Answer from the drawing. Dimensions are ordinates in mm from the lowest x, y and z of the part. Coordinates: 2 decimals unless noted, no trailing zeros. Write each loop counter-clockwise with the first axis right and the second up, starting at its lowest first coordinate (ties: lowest second). Pieces come first, ordered by that corner, then holes. Notation, with made-up numbers: M 17.5,69 L 39.5,69 A15 cw 39.5,85 Z; hole C 49,34.25 d6. An arc over 180 degrees is marked long. Put each result on its own line as item: value. Start each with the question number.
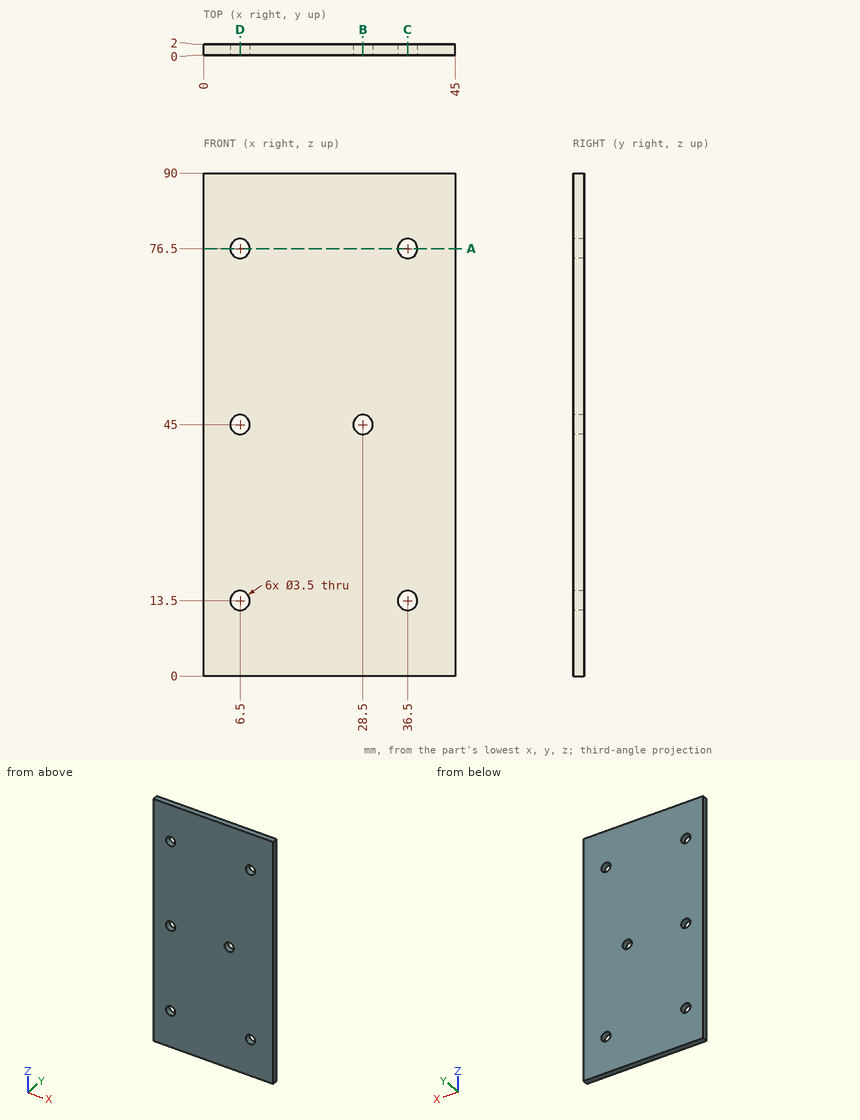
1) Straight lines are drawn through the part: probe 1 along Z at (x, y) = (6.5, 1.25); probe 2 along Z at (x, y) = (36.5, 0.3); probe 3 along X at (y, z) = (1.2, 76.5). For each, find the intervals that lie inside material, in ascending order.
2) A cutting plane is placed at D-D on x = 6.5. Write down the section's boundary in (y, z).
3) A cutting plane is placed at C-C on x = 36.5. Write down the section's boundary in (y, z), then the cut area to 3 significant figures.
4) A cutting plane is placed at A-A on z = 76.5. Write down the section's boundary in (x, y), then the cut area to 3 significant figures.
5) A cutting plane is placed at B-B on x = 28.5. Write down the section's boundary in (y, z), then the cut area to 3 significant figures.
Answers follow:
1. probe 1: z = 0 to 11.75, 15.25 to 43.25, 46.75 to 74.75, 78.25 to 90
1. probe 2: z = 0 to 11.75, 15.25 to 74.75, 78.25 to 90
1. probe 3: x = 0 to 4.75, 8.25 to 34.75, 38.25 to 45
2. outline: M 0,0 L 2,0 L 2,11.75 L 0,11.75 Z; M 0,15.25 L 2,15.25 L 2,43.25 L 0,43.25 Z; M 0,46.75 L 2,46.75 L 2,74.75 L 0,74.75 Z; M 0,78.25 L 2,78.25 L 2,90 L 0,90 Z
3. outline: M 0,0 L 2,0 L 2,11.75 L 0,11.75 Z; M 0,15.25 L 2,15.25 L 2,74.75 L 0,74.75 Z; M 0,78.25 L 2,78.25 L 2,90 L 0,90 Z
3. area: 166 mm²
4. outline: M 0,0 L 4.75,0 L 4.75,2 L 0,2 Z; M 8.25,0 L 34.75,0 L 34.75,2 L 8.25,2 Z; M 38.25,0 L 45,0 L 45,2 L 38.25,2 Z
4. area: 76.0 mm²
5. outline: M 0,0 L 2,0 L 2,43.25 L 0,43.25 Z; M 0,46.75 L 2,46.75 L 2,90 L 0,90 Z
5. area: 173 mm²
